Read the model definition and answer for the solid it produces. Units are mm, in the model's axes. Face numbers are marked on the shaded views. A direction names the side the tool comes from. Give positions to 0.01 mm unless a question says otherwise; leave off trailing zeros. Loops run counter-clockwise (first coordinate to the right, second up) from the corner with the lowest first, then second, coordinate; pieces in that order, holes last. Notation, with made-up numbers: (22.25, 48.5) - (76.25, 48.5) arc R13 cw to (76.25, 59.5) - close; hole circle Ø3 at (0.5, -35). An arc over 180 degrees is marked (long way). Write each question's results on one line, items separated by ' | '. Start each with the question number.
Q1. Given pin 1 (13.5 mm diameter, centred on x = 6, y = 2.5, fed in from +Z); pin 2 (8 mm diameter, centred on x = 11.5, y = -4.5, fed in from -Z), each flat-ended and moving along its own axis, determine where each tip first touches the part or whether it passes through.
Q2. For the marked faces 1, 2 and 3, determine the directions among +Z, -Z, +X, -X, +Y, -Y from which every point of the face is accessible in a straight line to the end or side of a thin tool.
Q3. Find the intervals of material crossed by line 1 (Z direction, x = -6, y = 9); line 2 (X direction, y = 4, z = 0.5); line 3 (X direction, y = 3.5, z = 9.5), in increasing order. Write a range as from..to.
Q4. The part is cut by section D-D, the plane x = -32. Write down the section's boundary in (y, z) (3 decimals), plus the area to 3 significant figures.
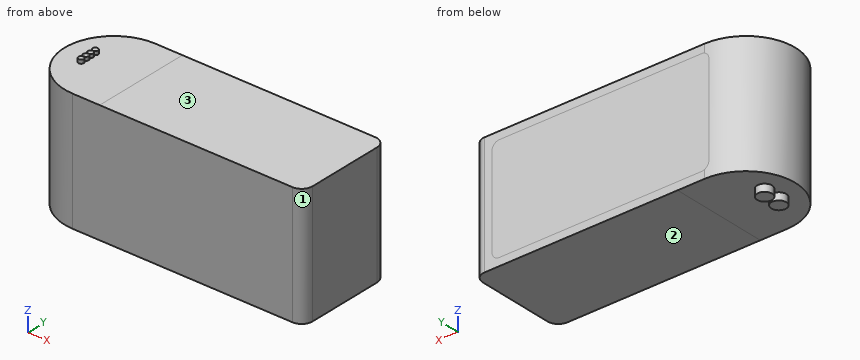
```python
from build123d import *

# Parameters (mm, degrees)
ESBO_O1_W                = 77
ESBO_O1_H                = 33
RESSALTO_EXTRUS_O1_DEPTH = 13.55
FILETE1_RADIUS           = 13.55
FILETE1_LENGTH           = 33
FILETE2_R                = 3
ESBO_O2_R                = 0.75
RESSALTO_EXTRUS_O6_DEPTH = 1
ESBO_O3_R                = 2.05
RESSALTO_EXTRUS_O7_DEPTH = 2
RESSALTO_EXTRUS_O8_DEPTH = 0.001
RESSALTO_EXTRUS_O9_DEPTH = 0.0001


with BuildPart() as part:
    # Esboço1 → Ressalto-extrusão1 (new, symmetric)
    with BuildSketch(Plane(origin=(0, 0, 0), x_dir=(1, 0, 0), z_dir=(0, 1, 0))):
        Rectangle(ESBO_O1_W, ESBO_O1_H)
    extrude(amount=RESSALTO_EXTRUS_O1_DEPTH, both=True)

    # Filete1: full round fillet: the end face becomes a half cylinder, R = half its width
    filete1_face = Plane((-38.5, 0, 0), x_dir=(0, 0, -1), z_dir=(-1, 0, 0))  # on the end face: x along it, z out of the body
    filete1_slab = filete1_face.offset(-FILETE1_RADIUS / 2) * Box(FILETE1_LENGTH, 2 * FILETE1_RADIUS, FILETE1_RADIUS, mode=Mode.PRIVATE)  # the body's end, R deep
    filete1_round = Plane((-24.95, 0, 0), x_dir=(-1, 0, 0), z_dir=(0, 0, -1)) * Cylinder(FILETE1_RADIUS, FILETE1_LENGTH, mode=Mode.PRIVATE)  # its axis R under the face
    add(filete1_slab - filete1_round, mode=Mode.SUBTRACT)

    # Filete2
    filete2_edges = [part.edges().sort_by_distance(p)[0] for p in [
        (38.5, 13.55, 0),
        (38.5, -13.55, 0),
    ]]
    fillet(filete2_edges, radius=FILETE2_R)

    # Esboço2 → Ressalto-extrusão6 (add)
    with BuildSketch(Plane.XY.offset(16.5)):
        with Locations(Location((-32, 2.325, 0), (0, 0, 180))):
            Circle(ESBO_O2_R)
        with Locations(Location((-32, 0.775, 0), (0, 0, 180))):
            Circle(ESBO_O2_R)
        with Locations(Location((-32, -0.775, 0), (0, 0, 180))):
            Circle(ESBO_O2_R)
        with Locations(Location((-32, -2.325, 0), (0, 0, 180))):
            Circle(ESBO_O2_R)
    extrude(amount=RESSALTO_EXTRUS_O6_DEPTH)

    # Esboço3 → Ressalto-extrusão7 (add)
    with BuildSketch(Plane(origin=(0, 0, -16.5), x_dir=(-1, 0, 0), z_dir=(0, 0, -1))):
        with Locations(Location((32, 2.325, 0), (0, 0, 180))):
            Circle(ESBO_O3_R)
        with Locations(Location((32, -2.325, 0), (0, 0, 180))):
            Circle(ESBO_O3_R)
    extrude(amount=RESSALTO_EXTRUS_O7_DEPTH)

    # Esboço4 → Ressalto-extrusão8 (add)
    with BuildSketch(Plane.XY.offset(16.5)):
        with BuildLine():
            Line((-17.5, -13.55), (-17.5, 13.55))
            Line((-17.5, 13.55), (-24.95, 13.55))
            ThreePointArc((-24.95, 13.55), (-38.5, 0), (-24.95, -13.55))
            Line((-24.95, -13.55), (-17.5, -13.55))
        make_face()
    ressalto_extrus_o8 = extrude(amount=RESSALTO_EXTRUS_O8_DEPTH)

    # Espelhar1: Ressalto-extrusão8 across plane
    add(ressalto_extrus_o8.mirror(Plane.XY))

    # Esboço6 → Ressalto-extrusão9 (add)
    with BuildSketch(Plane(origin=(0, 13.55, 0), x_dir=(1, 0, 0), z_dir=(0, 1, 0))):
        with BuildLine():
            Line((-24.12, 14.381), (31.5, 14.381))
            ThreePointArc((31.5, 14.381), (32.914213562, 13.795213562), (33.5, 12.381))
            Line((33.5, 12.381), (33.5, -12.381))
            ThreePointArc((33.5, -12.381), (32.914213562, -13.795213562), (31.5, -14.381))
            Line((31.5, -14.381), (-24.12, -14.381))
            ThreePointArc((-24.12, -14.381), (-25.534213562, -13.795213562), (-26.12, -12.381))
            Line((-26.12, -12.381), (-26.12, 12.381))
            ThreePointArc((-26.12, 12.381), (-25.534213562, 13.795213562), (-24.12, 14.381))
        make_face()
    extrude(amount=RESSALTO_EXTRUS_O9_DEPTH)


solid = part.part
```
Check sheet entries:
1) pin 1: stops at z = 16.5 | pin 2: stops at z = -16.5
2) face 1: +Z, -Z, +X, -Y | face 2: -Z, +X, +Y, -Y | face 3: +Z, +X, +Y, -Y
3) line 1: z = -16.5..16.5 | line 2: x = -37.9..38.5 | line 3: x = -38.04..38.5
4) outline: (-11.572, -16.501) - (-4.375, -16.501) - (-4.375, -18.5) - (-0.275, -18.5) - (-0.275, -16.501) - (0.275, -16.501) - (0.275, -18.5) - (4.375, -18.5) - (4.375, -16.501) - (11.572, -16.501) - (11.572, 16.501) - (3.075, 16.501) - (3.075, 17.5) - (1.575, 17.5) - (1.575, 16.501) - (1.525, 16.501) - (1.525, 17.5) - (0.025, 17.5) - (0.025, 16.501) - (-0.025, 16.501) - (-0.025, 17.5) - (-1.525, 17.5) - (-1.525, 16.501) - (-1.575, 16.501) - (-1.575, 17.5) - (-3.075, 17.5) - (-3.075, 16.501) - (-11.572, 16.501) - close | area: 786 mm^2
